```python
from build123d import *

# Parameters (mm, degrees)
BOSS_EXTRUDE1_DEPTH      = 3.25
BOSS_EXTRUDE1_DEPTH_BACK = 3.25
SKETCH1_W                = 10
SKETCH1_H                = 0.5
SKETCH1_W_2              = 28
SKETCH1_H_2              = 16
SKETCH1_R                = 1.75
BOSS_EXTRUDE2_DEPTH      = 1.5
BOSS_EXTRUDE2_DEPTH_BACK = 8
SKETCH2_W                = 28
SKETCH2_H                = 16
SKETCH2_R                = 1.75
CUT_EXTRUDE1_DEPTH       = 9.5
CUT_EXTRUDE2_DEPTH       = 1.5
FILLET1_R                = 1
FILLET2_R                = 1
FILLET3_R                = 3


with BuildPart() as part:
    # Sketch1 → Boss-Extrude1 (new, two sides: drawn at the far end of the back side and taken through both)
    # profile 1 of 4: a face of its own
    with BuildSketch(Plane.XY.offset(-BOSS_EXTRUDE1_DEPTH_BACK)):
        with Locations((-5, 6.25)):
            Rectangle(SKETCH1_W, SKETCH1_H)
    # profile 2 of 4: a face of its own
    with BuildSketch(Plane.XY.offset(-BOSS_EXTRUDE1_DEPTH_BACK)):
        with Locations((-5, 11.75)):
            Rectangle(SKETCH1_W, SKETCH1_H)
    # profile 3 of 4: a face of its own
    with BuildSketch(Plane.XY.offset(-BOSS_EXTRUDE1_DEPTH_BACK)):
        with Locations((14, 8)):
            Rectangle(SKETCH1_W_2, SKETCH1_H_2)
        with Locations((2.75, 3.25)):
            Circle(SKETCH1_R, mode=Mode.SUBTRACT)
        with Locations((25.25, 13.25)):
            Circle(SKETCH1_R, mode=Mode.SUBTRACT)
    # profile 4 of 4: a face of its own
    with BuildSketch(Plane.XY.offset(-BOSS_EXTRUDE1_DEPTH_BACK)):
        with BuildLine():
            Line((13, 16), (13.7, 16))
            Line((13.7, 16), (13.7, 18.2))
            ThreePointArc((13.7, 18.2), (13.553553391, 18.553553391), (13.2, 18.7))
            Line((13.2, 18.7), (4, 18.7))
            Line((4, 18.7), (4, 18))
            Line((4, 18), (12.5, 18))
            ThreePointArc((12.5, 18), (12.853553391, 17.853553391), (13, 17.5))
            Line((13, 17.5), (13, 16))
        make_face()
    extrude(amount=BOSS_EXTRUDE1_DEPTH + BOSS_EXTRUDE1_DEPTH_BACK)

    # Sketch2 → Boss-Extrude2 (add, two sides: drawn at the far end of the back side and taken through both)
    with BuildSketch(Plane(origin=(0, 0, -3.25), x_dir=(-1, 0, 0), z_dir=(0, 0, -1)).offset(-BOSS_EXTRUDE2_DEPTH_BACK)):
        with Locations((-14, 8)):
            Rectangle(SKETCH2_W, SKETCH2_H)
        with Locations(Location((-25.25, 13.25, 0), (0, 0, 180))):
            Circle(SKETCH2_R, mode=Mode.SUBTRACT)
        with Locations(Location((-2.75, 3.25, 0), (0, 0, 180))):
            Circle(SKETCH2_R, mode=Mode.SUBTRACT)
    extrude(amount=BOSS_EXTRUDE2_DEPTH + BOSS_EXTRUDE2_DEPTH_BACK)

    # Sketch3 → Cut-Extrude1 (cut)
    with BuildSketch(Plane(origin=(0, 12, 0), x_dir=(1, 0, 0), z_dir=(0, 1, 0))):
        with BuildLine():
            ThreePointArc((-5.25, -1.25), (-4, 0), (-5.25, 1.25))
            add(Edge.make_bspline(
                [(-5.25, 1.25), (-8.75, 0), (-5.25, -1.25)],
                knots=[0.849927106, 0.849927106, 0.849927106, 1.849927106, 1.849927106, 1.849927106], degree=2))
        make_face()
    extrude(amount=-CUT_EXTRUDE1_DEPTH, mode=Mode.SUBTRACT)

    # Sketch4 → Cut-Extrude2 (cut)
    with BuildSketch(Plane(origin=(0, 18.7, 0), x_dir=(1, 0, 0), z_dir=(0, 1, 0))):
        with BuildLine():
            ThreePointArc((8.45, -1.25), (9.7, 0), (8.45, 1.25))
            add(Edge.make_bspline(
                [(8.45, 1.25), (4.95, 0), (8.45, -1.25)],
                knots=[0.849927106, 0.849927106, 0.849927106, 1.849927106, 1.849927106, 1.849927106], degree=2))
        make_face()
    extrude(amount=-CUT_EXTRUDE2_DEPTH, mode=Mode.SUBTRACT)

    # Fillet1
    fillet1_edges = [part.edges().sort_by_distance(p)[0] for p in [
        (-5.25, 6.25, 1.25),
        (-5.25, 6.25, -1.25),
        (-5.25, 11.75, 1.25),
        (-5.25, 11.75, -1.25),
        (8.45, 18.35, -1.25),
        (8.45, 18.35, 1.25),
    ]]
    fillet(fillet1_edges, radius=FILLET1_R)

    # Fillet2
    fillet2_edges = [part.edges().sort_by_distance(p)[0] for p in [
        (-10, 6.25, -3.25),
        (4, 18.35, -3.25),
        (-10, 6.25, 3.25),
        (-10, 11.75, 3.25),
        (4, 18.35, 3.25),
        (-10, 11.75, -3.25),
    ]]
    fillet(fillet2_edges, radius=FILLET2_R)

    # Fillet3
    fillet3_edges = [part.edges().sort_by_distance(p)[0] for p in [
        (0, 16, 0),
        (28, 16, 0),
        (28, 0, 0),
        (0, 0, 0),
    ]]
    fillet(fillet3_edges, radius=FILLET3_R)


solid = part.part
```
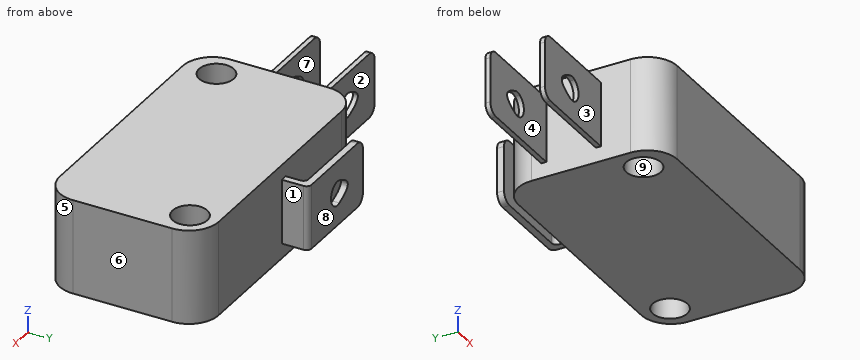
Design review of the part built by this model. Coordinates are the model's own, in mm. Face numbers are marked on the shaded views. A direction names the side the tool comes from. Coordinates: 2 decimals unless noted, no trailing zeros. Write each loop counter-clockwise with the first axis right and the second up, starting at its lowest first coordinate (ties: lowest second). Pieces come first, ordered by that corner, then holes.
1) Add section C-C (z = 0.25). State how many separate pieces and enclosed holes the cut face has, plus the area to 3 significant figures.
2) To check wall thickness, follow L1, parallel to X at y = 3.25, z = -2.25; L2, parallel to Y at x = 11, z = 2.25; L3, parallel to Y at x = -6.5, z = -2.5. State the ranges of each line that lie inside material, in increasing order.
3) Add section B-B (y = 2.5). Write out the cut boundary in (x, z).
4) Mouldability with a two-part tool opening along Y and no side actions: class the marked faces 6, 7, 8 and 9 as +Y half, -Y half, draft (parallel to the pull), parting line (faces both ways), or undercut.
5) Add section D-D (z = 2.75). Write out the cut boundary in (x, y).
6) Machinability: for the marked faces 1, 2, 3, 4 and 5, which of the approach directions +Z, -Z, +X, -X, +Y, -Y give a long, thin tool a straight path to every point of the face, cutting with its end or side? Answer none if there is none.
7) Add section A-A (x = -1). Write out the cut boundary in (y, z), plus the area to 3 significant figures.
8) Insertion check: pin 1 (2.5 mm diameter, centred on y = 16.5, z = 1.5, fed in from +X); pin 2 (3.5 mm diameter, centred on x = -7, z = 0.5, fed in from -Y); pin 3 (0.6 mm diameter, centred on x = -4, y = 12, fed in from -Z). Each pin has a flat end and moves straight along its axis. Give the tip position at first contact, or say it passes through.
Check result:
1. separate pieces: 4
1. enclosed holes: 2
1. area: 434 mm2
2. L1: x = 0 to 1, 4.5 to 28
2. L2: y = 0 to 16, 18 to 18.7
2. L3: y = 6 to 6.5, 11.5 to 12
3. outline: (0.04, -4.75) - (1.17, -4.75) - (1.17, 4.75) - (0.04, 4.75) - close; (4.33, -4.75) - (27.96, -4.75) - (27.96, 4.75) - (4.33, 4.75) - close
4. face 6: draft
4. face 7: undercut
4. face 8: +Y half
4. face 9: undercut
5. outline: (-9.87, 6) - (0, 6) - (0, 3) arc R3 ccw to (3, 0) - (25, 0) arc R3 ccw to (28, 3) - (28, 13) arc R3 ccw to (25, 16) - (13.7, 16) - (13.7, 18.2) arc R0.5 ccw to (13.2, 18.7) - (4.13, 18.7) - (4.13, 18) - (12.5, 18) arc R0.5 cw to (13, 17.5) - (13, 16) - (3, 16) arc R3 ccw to (0, 13) - (0, 12) - (-9.87, 12) - (-9.87, 11.5) - (0, 11.5) - (0, 6.5) - (-9.87, 6.5) - close; hole circle Ø3.5 at (2.75, 3.25); hole circle Ø3.5 at (25.25, 13.25)
6. face 1: +Z, -Z, +X, +Y
6. face 2: +Z, -Z, -X, +Y
6. face 3: +Z, -Z, -X, -Y
6. face 4: +Z, -Z, -X
6. face 5: +Z, -Z, +X, -Y
7. outline: (6, -3.25) - (6.5, -3.25) - (6.5, 3.25) - (6, 3.25) - close; (11.5, -3.25) - (12, -3.25) - (12, 3.25) - (11.5, 3.25) - close
7. area: 6.50 mm2
8. pin 1: stops at x = 26.98
8. pin 2: stops at y = 6
8. pin 3: stops at z = -3.25
